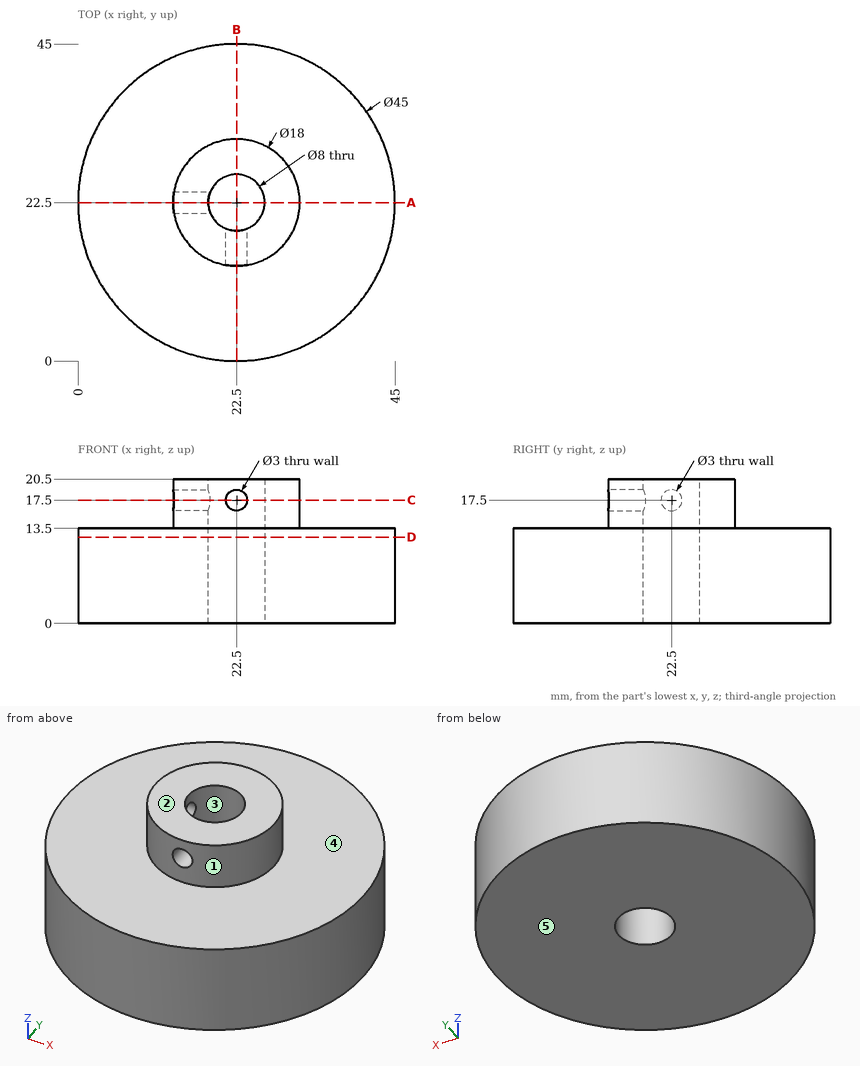
Verification items for this drawing (mm, ordinates from the low corner). A direction names the side the tool comes from. Give positions to 0.01 mm unless a question says otherwise; leave off trailing zeros. Loops run counter-clockwise (first coordinate to the right, second up) from the corner with the lowest first, then second, coordinate; pieces in that order, holes last. Notation, with made-up numbers: M -10.75,54.25 L -1.75,54.25 A7 cw -1.75,62.25 Z; hole C 67.25,20 d7. An arc over 180 degrees is marked long. Write item = value, one per line.
(1) Sectioned sample at C-C, the plane z = 17.5. Record the cut outline in (x, y).
Answer below:
outline = M 13.63,21 A9 ccw 21,13.63 L 21,18.79 A4 cw 18.79,21 Z; M 13.63,24 L 18.79,24 A4 cw long 24,18.79 L 24,13.63 A9 ccw long Z
(2) Sectioned sample at D-D, the plane z = 12.25. Record the cut outline in (x, y).
Answer below:
outline = C 22.5,22.5 d45; hole C 22.5,22.5 d8
(3) Tool access check on the marked faces 4 and 5. Record the directions out of +Z, -Z, +X, -X, +Y, -Y that give a thin tool (end or side, any length) a straight path to the whole face; none if there is none.
Answer below:
face_4 = +Z
face_5 = -Z, +X, -X, +Y, -Y
(4) Release check for a two-part mould opening along Y. For the marked faces 1, 2 and 3 record: released by +Y, released by -Y, zero draft, split by the parting line, or undercut.
Answer below:
face_1 = split by the parting line
face_2 = zero draft
face_3 = undercut
(5) Gauge pin test, flat ends, axial feed: pin 1 Ø10 at (x, y) = (10, 10.5) entering from +Z; pin 2 Ø12 at (x, z) = (15, 7.5) entering from -Y; pin 3 Ø4 at (x, z) = (22.5, 17.5) entering from -Y. Record the tip position at first contact, or that the pin passes through.
Answer below:
pin_1 = 13.5
pin_2 = 0.05
pin_3 = 13.5
(6) Sectioned sample at A-A, the plane y = 22.5. Record the cut outline in (x, z).
Answer below:
outline = M 0,0 L 18.5,0 L 18.5,16 L 13.5,16 L 13.5,13.5 L 0,13.5 Z; M 13.5,19 L 18.5,19 L 18.5,20.5 L 13.5,20.5 Z; M 26.5,0 L 45,0 L 45,13.5 L 31.5,13.5 L 31.5,20.5 L 26.5,20.5 Z
(7) Material ranges on line 1 (Z direction, x = 21, y = 40); line 2 (X direction, y = 22.5, z = 14.5); line 3 (X direction, y = 17.5, z = 17.5), recorded low to high. Write a range as [from, to].
Answer below:
line_1 = [0, 13.5]
line_2 = [13.5, 18.5], [26.5, 31.5]
line_3 = [15.02, 21], [24, 29.98]
